CAD build for the part. Positions are in the model's coordinates, mm. Face numbers are marked on the shaded views. A direction names the side the tool comes from. Round coordinates to 2 decimals unless told otherwise and drop trailing zeros. Loops run counter-clockwise (first coordinate to the right, second up) from the corner with the lowest first, then second, coordinate; pieces in that order, holes last.
from build123d import *

# Parameters (mm, degrees)
SKETCH2_R           = 15
SKETCH2_R_2         = 11
BOSS_EXTRUDE1_DEPTH = 4
SKETCH3_R           = 15
SKETCH3_R_2         = 4
BOSS_EXTRUDE2_DEPTH = 8
BOSS_EXTRUDE5_DEPTH = 12
SKETCH7_R           = 3
CUT_EXTRUDE1_DEPTH  = 14


with BuildPart() as part:
    # Sketch2 → Boss-Extrude1 (new body)
    with BuildSketch(Plane.XY):
        Circle(SKETCH2_R)
        Circle(SKETCH2_R_2, mode=Mode.SUBTRACT)
    extrude(amount=BOSS_EXTRUDE1_DEPTH)

    # Sketch3 → Boss-Extrude2 (add)
    with BuildSketch(Plane.XY.offset(4)):
        Circle(SKETCH3_R)
        Circle(SKETCH3_R_2, mode=Mode.SUBTRACT)
    extrude(amount=BOSS_EXTRUDE2_DEPTH)

    # Sketch6 → Boss-Extrude5 (add)
    with BuildSketch(Plane.XY.offset(12)):
        with BuildLine():
            Line((-15, 0), (-15, -33))
            Line((-15, -33), (15, -33))
            Line((15, -33), (15, 0))
            ThreePointArc((15, 0), (0, -15), (-15, 0))
        make_face()
    extrude(amount=-BOSS_EXTRUDE5_DEPTH)

    # Sketch7 → Cut-Extrude1 (cut)
    with BuildSketch(Plane.XZ.offset(33)):
        with Locations((7, 6)):
            Circle(SKETCH7_R)
        with Locations((-7, 6)):
            Circle(SKETCH7_R)
    extrude(amount=-CUT_EXTRUDE1_DEPTH, mode=Mode.SUBTRACT)


solid = part.part
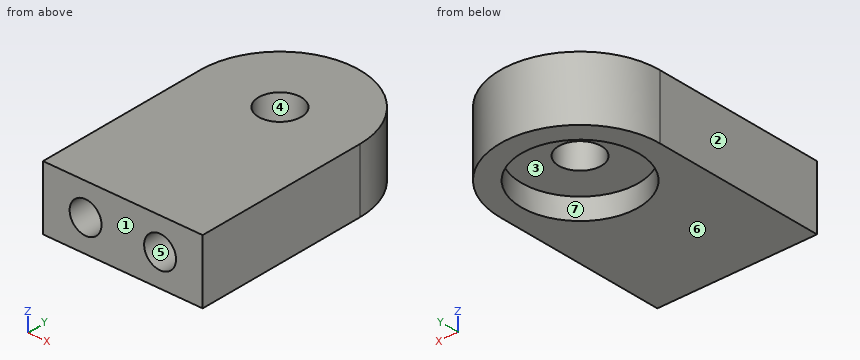
Item 1: Cut at D-D (y = -1). List the corners of the cut face in (x, z).
Verdict:
outline: (-15, 0) - (-10.95, 0) - (-10.95, 4) - (-3.87, 4) - (-3.87, 12) - (-15, 12) - close; (3.87, 4) - (10.95, 4) - (10.95, 0) - (15, 0) - (15, 12) - (3.87, 12) - close
Item 2: Flat gauge pins, fed straight in: P1, Ø8, axis at x = 9.5, y = -19.5, coming from the -Z side; P2, Ø1.5, axis at y = 3, z = 4, coming from the -X side; P3, Ø2, axis at y = 7, z = 4.5, coming from the -X side; P4, Ø3, axis at x = 11.5, z = 8.5, coming from the +Y side. Where does each tip first touch, or does it go through?
Verdict:
P1: stops at z = 0
P2: stops at x = -14.83
P3: stops at x = -13.75
P4: stops at y = 11.18
Item 3: Cut at A-A (x = 0). List the corners of the cut face in (y, z), plus the area to 3 significant figures.
Verdict:
outline: (-33, 0) - (-11, 0) - (-11, 4) - (-4, 4) - (-4, 12) - (-33, 12) - close; (4, 4) - (11, 4) - (11, 0) - (15, 0) - (15, 12) - (4, 12) - close
area: 424 mm2
Item 4: Wall check: L1, parallel to X at y = -25, z = 6.25; L2, parallel to Y at x = 0, z = 2.3; L3, parallel to Z at x = -7, y = -27.5. Give the ranges that are in metal, low to high.
Verdict:
L1: x = -15 to -9.99, -4.01 to 4.01, 9.99 to 15
L2: y = -33 to -11, 11 to 15
L3: z = 0 to 3, 9 to 12
Item 5: Cut at B-B (z = 6). List the corners of the cut face in (x, y).
Verdict:
outline: (-15, -33) - (-10, -33) - (-10, -19) - (-4, -19) - (-4, -33) - (4, -33) - (4, -19) - (10, -19) - (10, -33) - (15, -33) - (15, 0) arc R15 ccw to (-15, 0) - close; hole circle Ø8 at (0, 0)
Item 6: 3-axis set-ups, long thin cutter, end or side, ignore diameter. For the marked faces 5, 6 and 7: which of +Z, -Z, +X, -X, +Y, -Y reach the whole face in a straight line?
Verdict:
face 5: -Y
face 6: -Z, +X, -X, +Y, -Y
face 7: -Z
Item 7: Mould opens along Y. For the marked faces 1, 2, 3 and 4 say: released by +Y, released by -Y, zero draft, split by the parting line, or undercut.
Verdict:
face 1: released by -Y
face 2: zero draft
face 3: undercut
face 4: undercut
Item 8: Cut at C-C (y = -25.5). List the corners of the cut face in (x, z), plus the area to 3 significant figures.
Verdict:
outline: (-15, 0) - (15, 0) - (15, 12) - (-15, 12) - close; hole circle Ø6 at (-7, 6); hole circle Ø6 at (7, 6)
area: 303 mm2
